Drawing for the job (mm, zero at the part's lowest x, y, z). Give positions to 0.01 mm unless a question says otherwise; leave off trailing zeros. Order: outer loops, then holes, each group sorted by start corner. A loop starts at its lowest first (then second) coordinate and runs counter-clockwise, first axis right, second up. Notation, with made-up numbers: (-17, 62.25) - (28, 62.25) arc R21 ccw to (28, 84.25) - close; hole circle Ø7 at (54, 1.5). An arc over 180 degrees is marked (long way). Use a Markdown table: item, result.
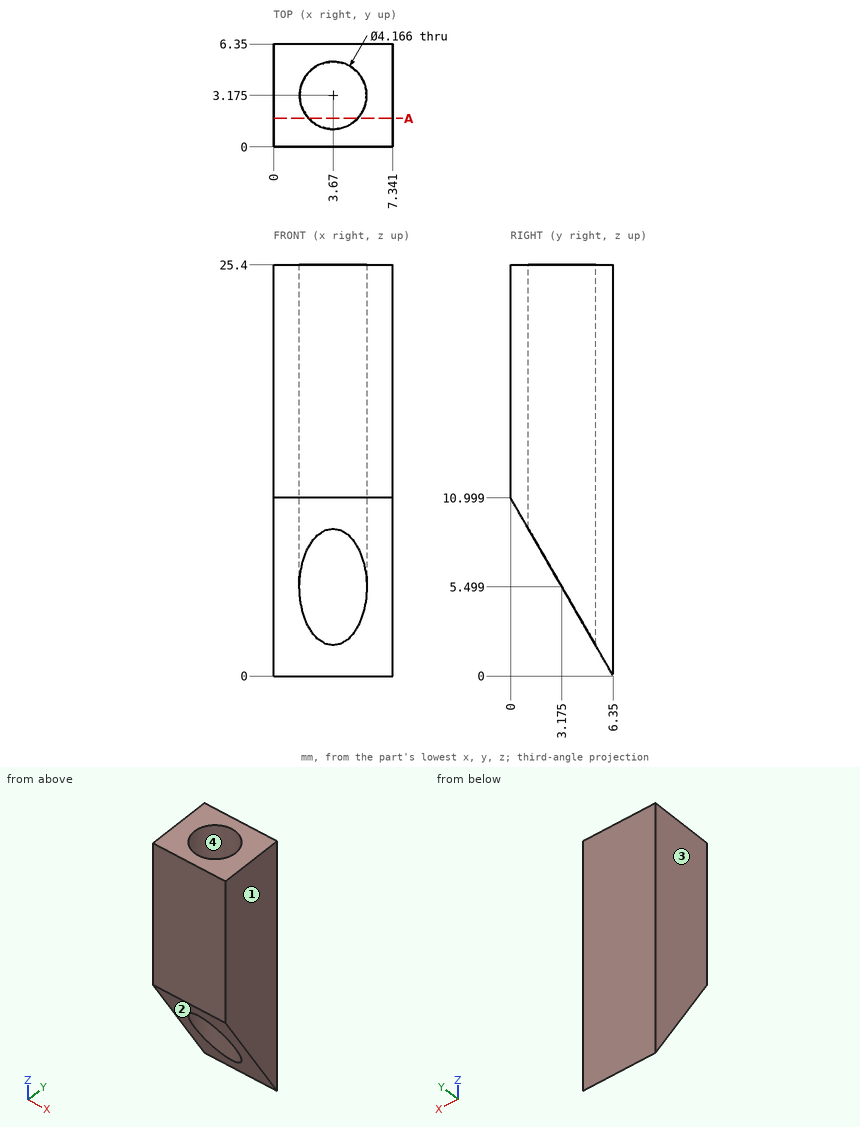
1) Pin check, flat tips, straight feed: P1, Ø3, axis at x = 2.5, y = 5, coming from the -Z side; P2, Ø1, axis at x = 5.5, y = 2, coming from the -Z side. Stop position of each tip, or through.
Computed:
| item | result |
|---|---|
| P1 | stops at z = 0 |
| P2 | stops at z = 6.7 |
2) Wall check: line 1 (Y direction, x = 3.75, z = 15.75); line 2 (Y direction, x = 2.5, z = 13.25); line 3 (X direction, y = 1.75, z = 23). Give the ranges that are in metal, low to high. Write a range as from..to.
Computed:
| item | result |
|---|---|
| line 1 | y = 0..1.09, 5.26..6.35 |
| line 2 | y = 0..1.45, 4.9..6.35 |
| line 3 | x = 0..2.15, 5.19..7.34 |
3) Slice it at A-A (y = 1.75). Write the cut outline in (x, z).
Computed:
| item | result |
|---|---|
| outline | (0, 7.97) - (2.15, 7.97) - (2.15, 25.4) - (0, 25.4) - close; (5.19, 7.97) - (7.34, 7.97) - (7.34, 25.4) - (5.19, 25.4) - close |
4) Two-plate mould, pull along X, no slides. Class the marked faces 1, 2, 3 and 4: +X half, -X half, draft (parallel to the pull), parting line (faces both ways), or undercut.
Computed:
| item | result |
|---|---|
| face 1 | +X half |
| face 2 | draft |
| face 3 | -X half |
| face 4 | undercut |
